Here's how the part is built. I have some questions about the finished solid (model axes, mm). Face numbers are marked on the shaded views. A direction names the side the tool comes from. Coordinates: 2 decimals unless noted, no trailing zeros. Loops run counter-clockwise (first coordinate to the right, second up) from the corner with the lowest first, then second, coordinate; pieces in that order, holes last. Notation, with made-up numbers: (-18, 77) -> (19, 77) arc R20 cw to (19, 95) -> close; hole circle Ø3 at (-29, 78). An arc over 180 degrees is marked (long way). Answer as a JSON object with one key per item and string values. Group by question number.
Q1. Thinking about a two-plate mould opening in Z: for the marked faces 1, 2, 3 and 4, which applies, released by +Z, released by -Z, zero draft, split by the parting line, or undercut?
Q2. On a 3-axis mill with a long thin cutter (end or side, diameter ignored), from which of +Z, -Z, +X, -X, +Y, -Y can I reach the whole of each face in a straight line? I mean the marked faces 5 and 6. Say none if no direction works.
Q3. I need wall thicknesses on line 1 (Z direction, x = 29, y = 0); line 2 (X direction, y = -24, z = -3); line 3 (Y direction, x = 12.5, z = -16.5). Which ranges of each line are inside material? Lowest first, please.
Q4. I want a section at B-B on x = 12. Write out the boundary of the cut face in (y, z), then the cut area to 3 significant figures.
Q5. I want a section at A-A on y = 0. Write out the boundary of the cut face in (x, z).
Q6. I want a section at D-D on x = -66. Write out the boundary of the cut face in (y, z), then the cut area to 3 significant figures.
Q7. I want a section at C-C on z = -6. Write out the boundary of the cut face in (x, y).
Q8. I'm going to push flat-ended pins straight in: pin 1 (1 mm diameter, centred on y = -39, z = -38, fed in from -X); pin 2 (6 mm diameter, centred on x = -73.5, y = -26, fed in from -Z). Where does each tip first touch, or does it pass through?
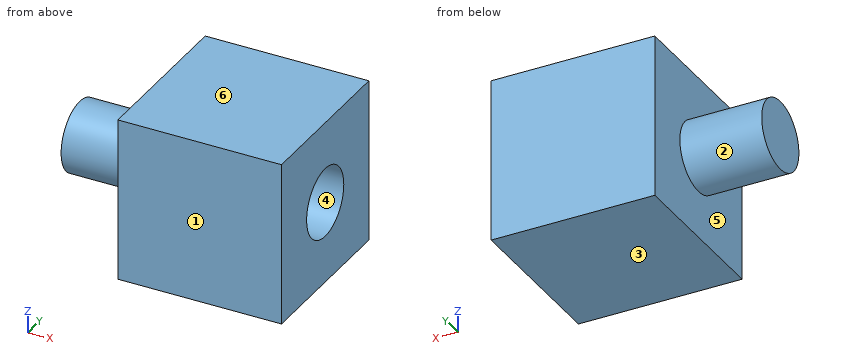
```python
from build123d import *

# Parameters (mm, degrees)
F1_W     = 101.6
F1_H     = 101.6
F2_DEPTH = 50.8
F3_R     = 21.6021439773
F4_DEPTH = 50.8
F5_R     = 21.6021439773
F6_DEPTH = 50.8


# Not quite as in the source:
# - a variable given as a bare number and used for a length is read in inches; the dataset says mm whatever the document's units were


with BuildPart() as f2:
    # F1 (on Front) → F2 (new body, symmetric)
    with BuildSketch(Plane.XZ):
        Rectangle(F1_W, F1_H)
    extrude(amount=F2_DEPTH, both=True)

    # F3 (on face) → F4 (cut)
    with BuildSketch(Plane.YZ.offset(50.8)):
        Circle(F3_R)
    extrude(amount=-F4_DEPTH, mode=Mode.SUBTRACT)

    # F5 (on face) → F6 (join)
    with BuildSketch(Plane(origin=(-50.8, 0, 0), x_dir=(0, -1, 0), z_dir=(-1, 0, 0))):
        Circle(F5_R)
    extrude(amount=F6_DEPTH)


solid = f2.part
```
Result set:
{
 "1": {"face 1": "zero draft", "face 2": "split by the parting line", "face 3": "released by -Z", "face 4": "undercut"},
 "2": {"face 5": "-X", "face 6": "+Z, +X, -X, +Y, -Y"},
 "3": {"line 1": "z = -50.8 to -21.6, 21.6 to 50.8", "line 2": "x = -50.8 to 50.8", "line 3": "y = -50.8 to -13.94, 13.94 to 50.8"},
 "4": {"outline": "(-50.8, -50.8) -> (50.8, -50.8) -> (50.8, 50.8) -> (-50.8, 50.8) -> close; hole circle Ø43.2 at (0, 0)", "area": "8,860 mm²"},
 "5": {"outline": "(-101.6, -21.6) -> (-50.8, -21.6) -> (-50.8, -50.8) -> (50.8, -50.8) -> (50.8, -21.6) -> (0, -21.6) -> (0, 21.6) -> (50.8, 21.6) -> (50.8, 50.8) -> (-50.8, 50.8) -> (-50.8, 21.6) -> (-101.6, 21.6) -> close"},
 "6": {"outline": "circle Ø43.2 at (0, 0)", "area": "1,470 mm²"},
 "7": {"outline": "(-101.6, -20.75) -> (-50.8, -20.75) -> (-50.8, -50.8) -> (50.8, -50.8) -> (50.8, -20.75) -> (0, -20.75) -> (0, 20.75) -> (50.8, 20.75) -> (50.8, 50.8) -> (-50.8, 50.8) -> (-50.8, 20.75) -> (-101.6, 20.75) -> close"},
 "8": {"pin 1": "stops at x = -50.8", "pin 2": "passes through"}
}
